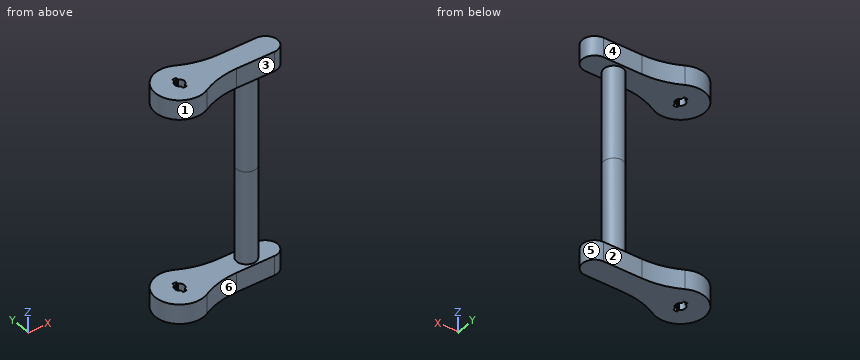
```python
from build123d import *

# Parameters (mm, degrees)
BOSS_EXTRUDE1_DEPTH = 20
SKETCH2_R           = 5
CUT_EXTRUDE1_DEPTH  = 20
CUT_EXTRUDE2_DEPTH  = 20
SKETCH6_R           = 10
BOSS_EXTRUDE2_DEPTH = 95


with BuildPart() as part:
    # Sketch1 → Boss-Extrude1 (new body)
    with BuildSketch(Plane.XY):
        with BuildLine():
            Line((90, 12.5), (50, 12.5))
            ThreePointArc((50, 12.5), (30.293980466, 14.925921863), (11.764705882, 22.058823529))
            ThreePointArc((11.764705882, 22.058823529), (-25, 0), (11.764705882, -22.058823529))
            ThreePointArc((11.764705882, -22.058823529), (30.293980466, -14.925921863), (50, -12.5))
            Line((50, -12.5), (90, -12.5))
            ThreePointArc((90, -12.5), (102.5, 0), (90, 12.5))
        make_face()
    extrude(amount=BOSS_EXTRUDE1_DEPTH)

    # Sketch2 → Cut-Extrude1 (cut)
    with BuildSketch(Plane.XY.offset(20)):
        Circle(SKETCH2_R)
    extrude(amount=-CUT_EXTRUDE1_DEPTH, mode=Mode.SUBTRACT)

    # Sketch5 → Cut-Extrude2 (cut)
    with BuildSketch(Plane.XY.offset(20)):
        with BuildLine():
            Line((-2, 7.228416147), (-2, -7.228416147))
            ThreePointArc((-2, -7.228416147), (0, -7.5), (2, -7.228416147))
            Line((2, -7.228416147), (2, 7.228416147))
            ThreePointArc((2, 7.228416147), (0, 7.5), (-2, 7.228416147))
        make_face()
    extrude(amount=-CUT_EXTRUDE2_DEPTH, mode=Mode.SUBTRACT)

    # Sketch6 → Boss-Extrude2 (add)
    with BuildSketch(Plane.XY.offset(20)):
        with Locations((70, 0)):
            Circle(SKETCH6_R)
    extrude(amount=BOSS_EXTRUDE2_DEPTH)

    # Mirror1: part across plane


with BuildPart() as part_1:
    add(part.part)
    add(part.part.mirror(Plane(origin=(70, 0, 115), x_dir=(1, 0, 0), z_dir=(0, 0, 1))))


solid = part_1.part
```
Part model, mm, in its own coordinate system. Face numbers are marked on the shaded views. A direction names the side the tool comes from. Give positions to 0.01 mm unless a question says otherwise; leave off trailing zeros. Loops run counter-clockwise (first coordinate to the right, second up) from the corner with the lowest first, then second, coordinate; pieces in that order, holes last. Notation, with made-up numbers: M 86.5,60.5 L 92.5,60.5 A30 ccw 92.5,91.5 Z; hole C 49.25,42.25 d3. An arc over 180 degrees is marked long. Return JSON: item names as keys, results as strings.
1) 3-axis set-ups, long thin cutter, end or side, ignore diameter. For the marked faces 1, 2 and 3: which of +Z, -Z, +X, -X, +Y, -Y reach the whole face in a straight line?
Calculated:
{"face 1": "+Z, -Z", "face 2": "+Z, -Z, +X, +Y", "face 3": "+Z, -Z, +X, -Y"}
2) Saw through at B-B, the plane x = 70. List the corners of the cut face in (y, z).
Calculated:
{"outline": "M -12.5,0 L 12.5,0 L 12.5,20 L 10,20 L 10,210 L 12.5,210 L 12.5,230 L -12.5,230 L -12.5,210 L -10,210 L -10,20 L -12.5,20 Z"}
3) Pull direction Y, two halves, no side cores. Call the marked faces 4, 5 and 6: released by +Y, released by -Y, zero draft, split by the parting line, or undercut.
Calculated:
{"face 4": "released by +Y", "face 5": "split by the parting line", "face 6": "released by -Y"}
4) Flat gauge pins, fed straight in: pin 1 Ø8 at (y, z) = (6.5, 144.5) entering from +X; pin 2 Ø16 at (x, z) = (71.5, 220.5) entering from -Y; pin 3 Ø1.3 at (y, z) = (-5.5, 217.5) entering from -X. Where does each tip first touch, or does it go through?
Calculated:
{"pin 1": "stops at x = 79.68", "pin 2": "stops at y = -12.5", "pin 3": "stops at x = -24.53"}
5) Saw through at C-C, the plane y = 17. List the corners of the cut face in (x, z).
Calculated:
{"outline": "M -18.33,0 L 23.34,0 L 23.34,20 L -18.33,20 Z; M -18.33,210 L 23.34,210 L 23.34,230 L -18.33,230 Z"}
6) Saw through at D-D, the plane x = 46.5. List the corners of the cut face in (y, z), then the cut area to 3 significant figures.
Calculated:
{"outline": "M -12.58,0 L 12.58,0 L 12.58,20 L -12.58,20 Z; M -12.58,210 L 12.58,210 L 12.58,230 L -12.58,230 Z", "area": "1,010 mm2"}
7) Saw through at A-A, the plane y = 0. List the corners of the cut face in (x, z).
Calculated:
{"outline": "M -25,0 L -5,0 L -5,20 L -25,20 Z; M -25,210 L -5,210 L -5,230 L -25,230 Z; M 5,0 L 102.5,0 L 102.5,20 L 80,20 L 80,210 L 102.5,210 L 102.5,230 L 5,230 L 5,210 L 60,210 L 60,20 L 5,20 Z"}
8) Drill centre lines: line 1 (Z direction, x = 39, y = 8.5); line 2 (Y direction, x = 89, z = 13); line 3 (X direction, y = -6.5, z = 214). Where is each one in solid material? Low to high.
Calculated:
{"line 1": "z = 0 to 20, 210 to 230", "line 2": "y = -12.5 to 12.5", "line 3": "x = -24.14 to -2, 2 to 100.68"}
